Can you work these out from the model? Positions are in its coordinate system, mm. A direction names the side the tool comes from. Coordinates: 2 decimals unless noted, no trailing zeros. Order: outer loops, then holes, each group sorted by start corner. A loop starts at its lowest first (then second) coordinate and runs counter-clockwise, first axis right, second up. Notation, with made-up numbers: (-33.75, -38) -> (2.25, -38) arc R18 cw to (2.25, -18) -> close; hole circle Ø4 at (54, 80.5). An arc over 180 degrees is marked (long way). Return JSON: item names as keys, results as strings. Group by question number.
1) Thinking about a two-plate mould opening in Y: for faces 3 (the cylindrical face through (-11.72, 16.7, 4.93)), 4 (the flat face through (-11.7, 3.8, 24.6)), 5 (the flat face through (-9, 13, 50)), 6 (the cylindrical face through (-15, 20, 25)), which applies, +Y half, -Y half, draft (parallel to the pull), parting line (faces both ways), or undercut?
2) If we section it at D-D, the plane z = 20: Please give me the cut outline in (x, y).
3) For faces 1 (the flat face through (-9, 13, 10)), 2 (the flat face through (-3.8, 12.7, 0)), which set-ups out of +Z, -Z, +X, -X, +Y, -Y let a thin tool reach every point of the face, with its end or its side?
4) If we section it at A-A, the plane x = -7.5: Please give me the cut outline in (y, z), then the cut area to 3 significant figures.
5) For pin 1 (6 mm diameter, centred on x = -14, y = 18, fed in from -Z); pin 2 (2 mm diameter, centred on x = -8, z = 9, fed in from -Y); pin 3 (1 mm diameter, centred on y = 9.5, z = 16.5, fed in from -X); pin 4 (5 mm diameter, centred on x = -12.5, z = 40.5, fed in from -Y), each with a flat end and sliding along its axis, tell me the tip position at first contact or that it passes through.
6) If I drill on probe 1 along X at (y, z) = (14.75, 3); probe 2 along X at (y, z) = (16.25, 4); probe 3 along Z at (x, y) = (-12, 16), over which ranges is the centre line in solid material (lowest first)? Write a range as from..to.
7) If we section it at B-B, the plane z = 4.5: Please give me the cut outline in (x, y).
8) If we section it at C-C, the plane y = 5.75: Please give me the cut outline in (x, z), then the cut area to 3 significant figures.
from build123d import *

# Parameters (mm, degrees)
SALIENTE_EXTRUIR1_DEPTH = 50
CROQUIS2_R              = 5
CORTAR_EXTRUIR1_DEPTH   = 10


with BuildPart() as part:
    # Croquis1 → Saliente-Extruir1 (new body)
    with BuildSketch(Plane.XY):
        with BuildLine():
            Line((0, 25), (0, 0))
            Line((0, 0), (-23.776412907, 7.725424859))
            ThreePointArc((-23.776412907, 7.725424859), (-14.694631307, 20.225424859), (0, 25))
        make_face()
    extrude(amount=SALIENTE_EXTRUIR1_DEPTH)

    # Croquis2 → Cortar-Extruir1 (cut)
    with BuildSketch(Plane(origin=(0, 0, 0), x_dir=(-1, 0, 0), z_dir=(0, 0, -1))):
        with Locations((9.035159756, 12.480979689)):
            Circle(CROQUIS2_R)
    extrude(amount=-CORTAR_EXTRUIR1_DEPTH, mode=Mode.SUBTRACT)


solid = part.part
Result sheet:
{
 "1": {"face 3": "undercut", "face 4": "-Y half", "face 5": "draft", "face 6": "+Y half"},
 "2": {"outline": "(-23.78, 7.73) -> (0, 0) -> (0, 25) arc R25 ccw to start"},
 "3": {"face 1": "-Z", "face 2": "-Z, +X, -X, +Y, -Y"},
 "4": {"outline": "(2.44, 0) -> (7.72, 0) -> (7.72, 10) -> (17.24, 10) -> (17.24, 0) -> (23.85, 0) -> (23.85, 50) -> (2.44, 50) -> close", "area": "975 mm2"},
 "5": {"pin 1": "stops at z = 0", "pin 2": "stops at y = 2.27", "pin 3": "stops at x = -23.32", "pin 4": "stops at y = 3.25"},
 "6": {"probe 1": "x = -20.19..-13.49, -4.58..0", "probe 2": "x = -19..-12.32, -5.75..0", "probe 3": "z = 10..50"},
 "7": {"outline": "(-23.78, 7.73) -> (0, 0) -> (0, 25) arc R25 ccw to start; hole circle Ø10 at (-9.04, 12.48)"},
 "8": {"outline": "(-17.7, 0) -> (0, 0) -> (0, 50) -> (-17.7, 50) -> close", "area": "885 mm2"}
}
